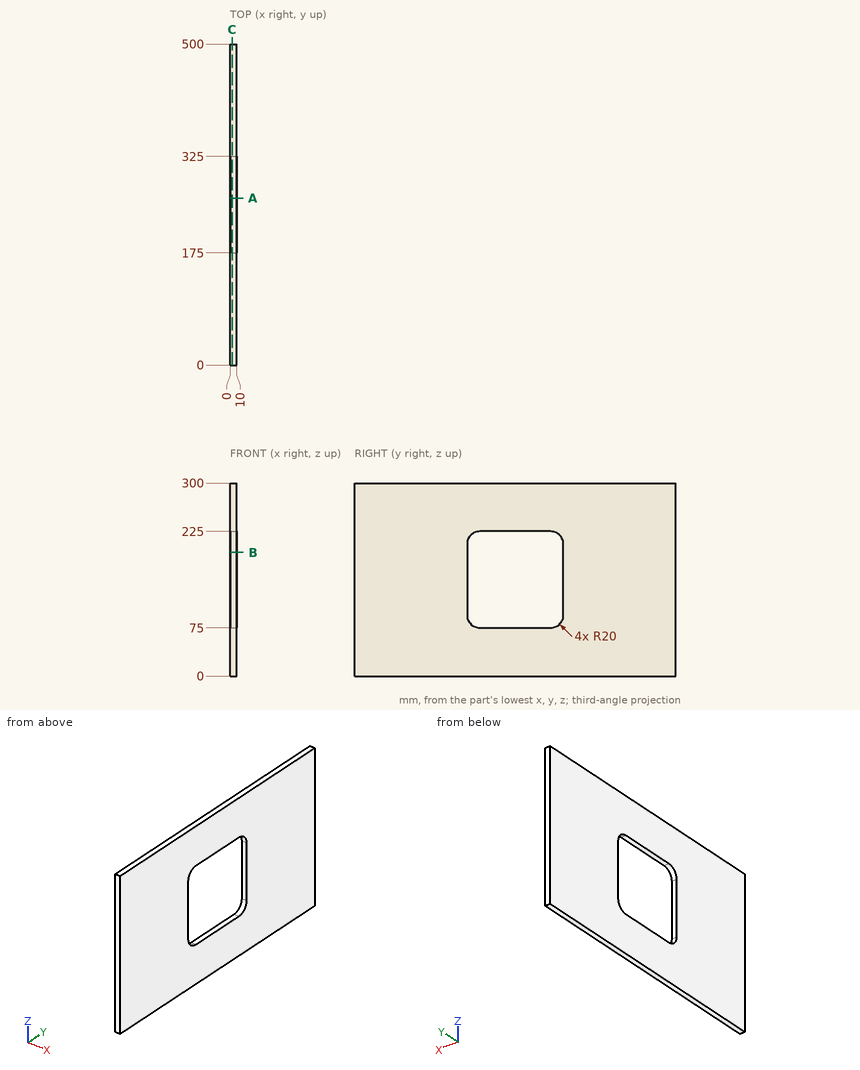
For this review, use the dimensioned drawing (mm, ordinates from the lowest corner) and the shaded views. Give positions to 0.01 mm unless a question says otherwise; leave off trailing zeros. Write each loop counter-clockwise with the first axis right and the second up, starting at its lowest first coordinate (ties: lowest second). Pieces come first, ordered by that corner, then holes.
(1) Consider section A-A, the plane y = 260. Give the boundary of the cut face in (x, z).
(2) Consider section C-C, the plane x = 3. Give the boundary of the cut face in (y, z).
(3) To check wall thickness, follow L1, parallel to Z at x = 7.25, y = 259.5; L2, parallel to Z at x = 0.5, y = 307; L3, parallel to Y at x = 3.5, z = 130. State the ranges of each line that lie inside material, in increasing order.
(4) Consider section B-B, the plane z = 192.5. Give the boundary of the cut face in (x, y).
(5) For P1, Ø2, axis at y = 265, z = 269, coming from the -X side, flat-tipped, find the tip position at first contact; note if it passes through.
Returned:
1. outline: (0, 0) - (10, 0) - (10, 75) - (0, 75) - close; (0, 225) - (10, 225) - (10, 300) - (0, 300) - close
2. outline: (0, 0) - (500, 0) - (500, 300) - (0, 300) - close; hole (175, 95) arc R20 ccw to (195, 75) - (305, 75) arc R20 ccw to (325, 95) - (325, 205) arc R20 ccw to (305, 225) - (195, 225) arc R20 ccw to (175, 205) - close
3. L1: z = 0 to 75, 225 to 300
3. L2: z = 0 to 75.1, 224.9 to 300
3. L3: y = 0 to 175, 325 to 500
4. outline: (0, 0) - (10, 0) - (10, 175) - (0, 175) - close; (0, 325) - (10, 325) - (10, 500) - (0, 500) - close
5. P1: stops at x = 0
